Answer from the drawing. Dimensions are ordinates in mm from the lowest x, y and z of the part. Coordinates: 2 decimals unless noted, no trailing zeros. Order: outer loops, then holes, each group sorted by start corner. A loop starts at its lowest first (then second) coordinate and runs counter-clockwise, first axis right, second up. Notation, with made-up numbers: M 28,64.25 L 53,64.25 A16 ccw 53,85.25 Z; hole C 62.25,69 d5. An arc over 180 degrees is marked long. One line per question, with ' | ' between items. Start each with the question number.
1) Given P1, Ø2.5, axis at x = 11, z = 111, coming from the +Y side; P2, Ø4, axis at x = 30, z = 119, coming from the -Y side; P3, Ø1.5, axis at y = 10, z = 151.5, coming from the -X side, each flat-ended and moving along its own axis, determine where each tip first touches the part or whether it passes through.
2) Consider probe 1 along X at (y, z) = (17.25, 117.5); probe 2 along Y at (x, z) = (3, 238.5); probe 3 along X at (y, z) = (11.5, 107). Determine where each line is inside the solid, lowest interval first.
3) Find section A-A, the plane z = 332. Write down the section's boundary in (x, y).
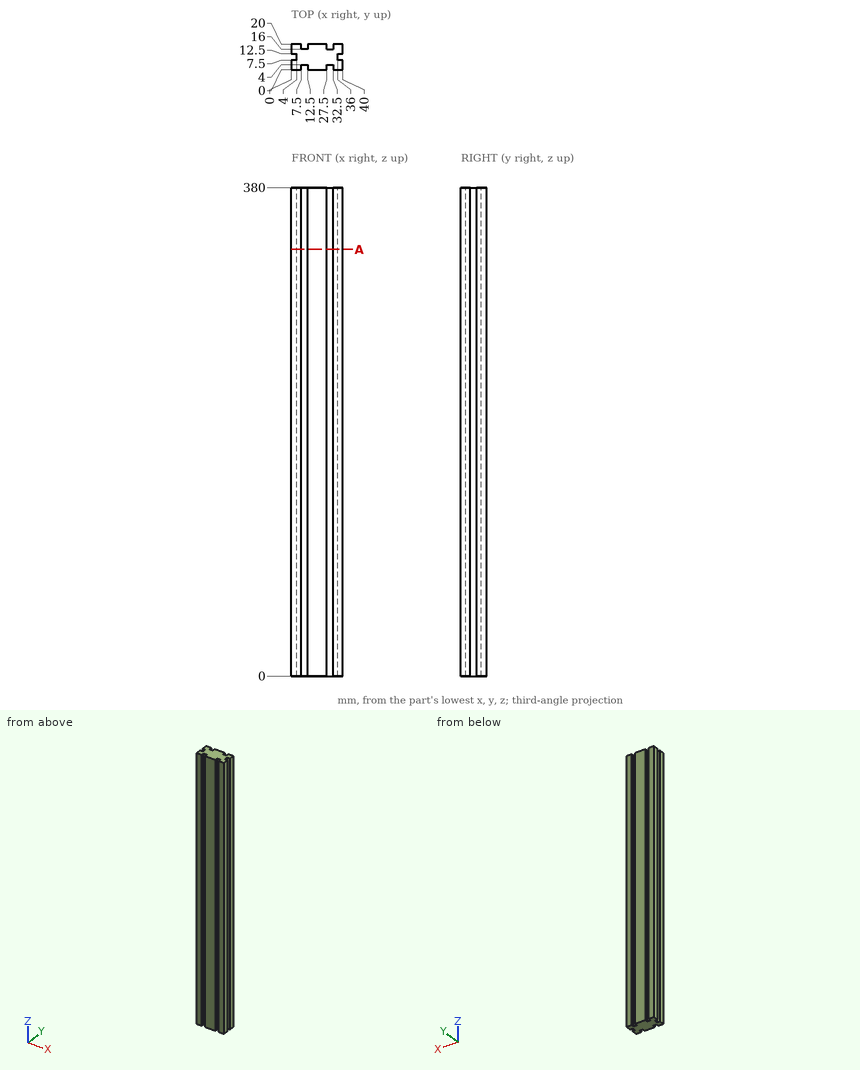
Report:
1) P1: stops at y = 16 | P2: stops at y = 4 | P3: stops at x = 4
2) probe 1: x = 0 to 7.5, 12.5 to 27.5, 32.5 to 40 | probe 2: y = 0 to 7.5, 12.5 to 20 | probe 3: x = 4 to 36
3) outline: M 0,0 L 7.5,0 L 7.5,4 L 12.5,4 L 12.5,0 L 27.5,0 L 27.5,4 L 32.5,4 L 32.5,0 L 40,0 L 40,7.5 L 36,7.5 L 36,12.5 L 40,12.5 L 40,20 L 32.5,20 L 32.5,16 L 27.5,16 L 27.5,20 L 12.5,20 L 12.5,16 L 7.5,16 L 7.5,20 L 0,20 L 0,12.5 L 4,12.5 L 4,7.5 L 0,7.5 Z
